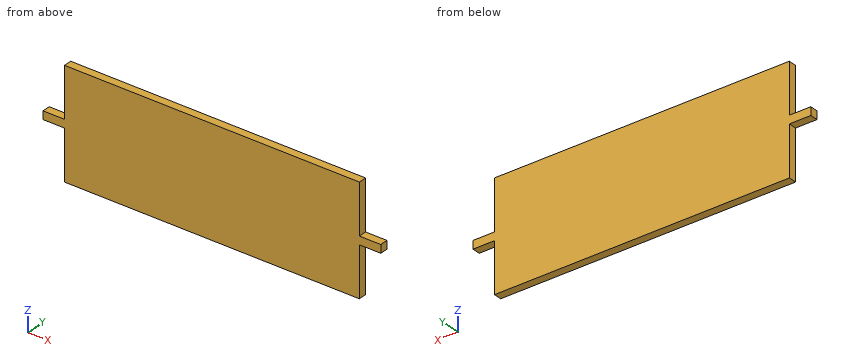
from build123d import *

# Parameters (mm, degrees)
SKETCH1_W           = 8
SKETCH1_H           = 1.5
SKETCH1_W_2         = 110
SKETCH1_H_2         = 18.5
BOSS_EXTRUDE1_DEPTH = 3


with BuildPart() as part:
    # Sketch1 → Boss-Extrude1 (new body)
    with BuildSketch(Plane(origin=(0, 0, 0), x_dir=(1, 0, 0), z_dir=(0, 1, 0))):
        with Locations((-4, 20.75)):
            Rectangle(SKETCH1_W, SKETCH1_H)
        with Locations((-4, 19.25)):
            Rectangle(SKETCH1_W, SKETCH1_H)
        Polygon((0, 20), (0, 18.5), (110, 18.5), (110, 20), (110, 21.5), (0, 21.5), align=None)
        with Locations((55, 30.75)):
            Rectangle(SKETCH1_W_2, SKETCH1_H_2)
        with Locations((55, 9.25)):
            Rectangle(SKETCH1_W_2, SKETCH1_H_2)
        with Locations((114, 20.75)):
            Rectangle(SKETCH1_W, SKETCH1_H)
        with Locations((114, 19.25)):
            Rectangle(SKETCH1_W, SKETCH1_H)
    extrude(amount=BOSS_EXTRUDE1_DEPTH)


solid = part.part
Read the model definition and answer for the solid it produces. Units are mm, in the model's axes. Coordinates: 2 decimals unless noted, no trailing zeros. Loops run counter-clockwise (first coordinate to the right, second up) from the corner with the lowest first, then second, coordinate; pieces in that order, holes last.
Q1. The part is cut by section B-B on z = -32. Write down the section's boundary in (x, y).
Q2. This flat-tipped pin is pushed along its axis until it touches: pin 1 Ø1.5 at (x, y) = (-5.5, 1) entering from +Z. Where does it stop, or does it pass through?
Q3. Consider probe 1 along X at (y, z) = (2, -27.5). Determine where the line is inside the solid, lowest interval first.
Q4. The part is cut by section A-A on y = 0.9. Write down the section's boundary in (x, z), and give its area (3 significant figures).
Results below:
1. outline: (0, 0) - (110, 0) - (110, 3) - (0, 3) - close
2. pin 1: stops at z = -18.5
3. probe 1: x = 0 to 110
4. outline: (-8, -21.5) - (0, -21.5) - (0, -40) - (110, -40) - (110, -21.5) - (118, -21.5) - (118, -18.5) - (110, -18.5) - (110, 0) - (0, 0) - (0, -18.5) - (-8, -18.5) - close
4. area: 4,450 mm2
